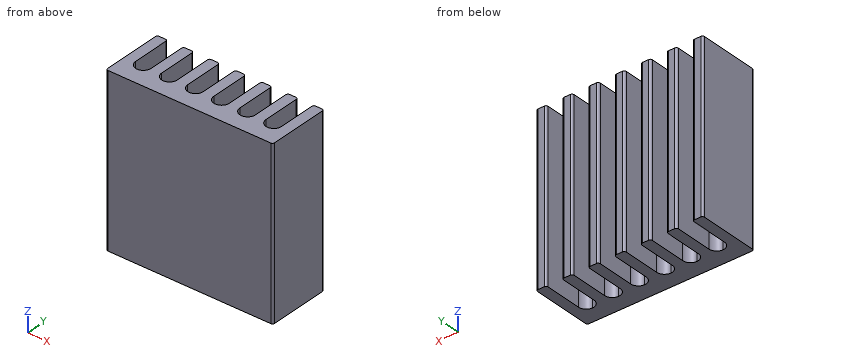
```python
from build123d import *

# Parameters (mm, degrees)
SKETCH2_W           = 16
SKETCH2_H           = 16
BOSS_EXTRUDE1_DEPTH = 1.5
SKETCH3_W           = 1
SKETCH3_H           = 4.5
BOSS_EXTRUDE2_DEPTH = 16
FILLET1_R           = 0.75
FILLET2_R           = 0.2


with BuildPart() as part:
    # Sketch2 → Boss-Extrude1 (new body)
    with BuildSketch(Plane(origin=(0, 0, 0), x_dir=(1, 0, 0), z_dir=(0, 1, 0))):
        Rectangle(SKETCH2_W, SKETCH2_H)
    extrude(amount=BOSS_EXTRUDE1_DEPTH)

    # Sketch3 → Boss-Extrude2 (add)
    with BuildSketch(Plane.XY.offset(8)):
        with Locations((-7.5, 3.75)):
            Rectangle(SKETCH3_W, SKETCH3_H)
        with Locations((-5, 3.75)):
            Rectangle(SKETCH3_W, SKETCH3_H)
        with Locations((-2.5, 3.75)):
            Rectangle(SKETCH3_W, SKETCH3_H)
        with Locations((0, 3.75)):
            Rectangle(SKETCH3_W, SKETCH3_H)
        with Locations((2.5, 3.75)):
            Rectangle(SKETCH3_W, SKETCH3_H)
        with Locations((5, 3.75)):
            Rectangle(SKETCH3_W, SKETCH3_H)
        with Locations((7.5, 3.75)):
            Rectangle(SKETCH3_W, SKETCH3_H)
    extrude(amount=-BOSS_EXTRUDE2_DEPTH)

    # Fillet1
    fillet1_edges = [part.edges().sort_by_distance(p)[0] for p in [
        (7, 1.5, 0),
        (5.5, 1.5, 0),
        (4.5, 1.5, 0),
        (3, 1.5, 0),
        (2, 1.5, 0),
        (0.5, 1.5, 0),
        (-0.5, 1.5, 0),
        (-2, 1.5, 0),
        (-3, 1.5, 0),
        (-4.5, 1.5, 0),
        (-5.5, 1.5, 0),
        (-7, 1.5, 0),
    ]]
    fillet(fillet1_edges, radius=FILLET1_R - 0.0001)  # a hair under: the kernel refuses the full size

    # Fillet2
    fillet2_edges = [part.edges().sort_by_distance(p)[0] for p in [
        (-7, 6, 0),
        (-8, 6, 0),
        (-4.5, 6, 0),
        (-5.5, 6, 0),
        (-2, 6, 0),
        (-3, 6, 0),
        (0.5, 6, 0),
        (-0.5, 6, 0),
        (-8, 0, 0),
        (3, 6, 0),
        (2, 6, 0),
        (5.5, 6, 0),
        (4.5, 6, 0),
        (8, 0, 0),
        (8, 6, 0),
        (7, 6, 0),
    ]]
    fillet(fillet2_edges, radius=FILLET2_R)


solid = part.part
```
Can you work these out from the model? Positions are in its coordinate system, mm. Round coordinates to 2 decimals unless told otherwise and drop trailing zeros. Loops run counter-clockwise (first coordinate to the right, second up) from the corner with the lowest first, then second, coordinate; pieces in that order, holes last. Notation, with made-up numbers: (86, 13) -> (135, 13) arc R13 ccw to (135, 26) -> close; hole circle Ø5 at (-37, 37). An arc over 180 degrees is marked (long way). Answer in a Markdown table with one row per item.
Item 1: Suppose I cut it at B-B, the plane x = 6. List the corners of the cut face in (y, z) for me.
Answer block:
| item | result |
|---|---|
| outline | (0, -8) -> (1.54, -8) -> (1.54, 8) -> (0, 8) -> close |
Item 2: If I drill on probe 1 along Y at (x, z) = (3.5, 1); probe 2 along Y at (x, z) = (1.75, 1.25), over which ranges is the centre line in solid material (lowest first)?
Answer block:
| item | result |
|---|---|
| probe 1 | 0 to 1.54 |
| probe 2 | 0 to 1.69 |
Item 3: Suppose I cut it at A-A, the plane y = 3.9. List the corners of the cut face in (x, z) for me, plus the area to 3 significant figures.
Answer block:
| item | result |
|---|---|
| outline | (-8, -8) -> (-7, -8) -> (-7, 8) -> (-8, 8) -> close; (-5.5, -8) -> (-4.5, -8) -> (-4.5, 8) -> (-5.5, 8) -> close; (-3, -8) -> (-2, -8) -> (-2, 8) -> (-3, 8) -> close; (-0.5, -8) -> (0.5, -8) -> (0.5, 8) -> (-0.5, 8) -> close; (2, -8) -> (3, -8) -> (3, 8) -> (2, 8) -> close; (4.5, -8) -> (5.5, -8) -> (5.5, 8) -> (4.5, 8) -> close; (7, -8) -> (8, -8) -> (8, 8) -> (7, 8) -> close |
| area | 112 mm² |
Item 4: Will this pin go through, and if not, where does the flat tip stop? P1, Ø2, axis at x = -2, z = 1.5, coming from the +Y side.
Answer block:
| item | result |
|---|---|
| P1 | y = 6 |
